The listing builds one solid part. Answer for the finished solid, in the listing's coordinates (mm). A direction names the side the tool comes from. Coordinates: 2 decimals unless noted, no trailing zeros. Order: outer loops, then holes, each group sorted by start corner. A loop starts at its lowest first (then second) coordinate and runs counter-clockwise, first axis right, second up. Notation, with made-up numbers: (80.25, -33) -> (119.25, -33) arc R9 cw to (119.25, -18) -> close; hole circle Ø10 at (83, 65). An arc over 180 degrees is marked (long way). Write item = value, one per line.
from build123d import *

# Parameters (mm, degrees)
SKETCH1_W               = 2.54
SKETCH1_H               = 6.35
SKETCH2_W               = 1.5875
SKETCH2_H               = 11.1125
CUT_EXTRUDE1_DEPTH      = 4.96875
CUT_EXTRUDE1_DEPTH_BACK = 4.96875


with BuildPart() as part:
    # Sketch1 → Revolve1 (revolve)
    with BuildSketch(Plane(origin=(0, 0, 0), x_dir=(0, 0, -1), z_dir=(1, 0, 0))):
        Polygon((0, 3.175), (0, 0), (3.96875, 0), (3.96875, 3.175), (2.54, 3.175), align=None)
        with Locations((1.27, 6.35)):
            Rectangle(SKETCH1_W, SKETCH1_H)
        Polygon((0, 14.2875), (0, 9.525), (2.54, 9.525), (3.175, 9.525), (1.5875, 14.2875), align=None)
    revolve(axis=Axis((0, 0, 0), (0, 1, 0)))

    # Sketch2 → Cut-Extrude1 (cut, two sides)
    with BuildSketch(Plane.XY) as cut_extrude1_sk:
        with Locations((0, 8.73125)):
            Rectangle(SKETCH2_W, SKETCH2_H)
    extrude(amount=CUT_EXTRUDE1_DEPTH, mode=Mode.SUBTRACT)
    extrude(cut_extrude1_sk.sketch, amount=-CUT_EXTRUDE1_DEPTH_BACK, mode=Mode.SUBTRACT)


solid = part.part
Q1. Each of these flat-tipped pins is pushed along its axis until it touches: pin 1 Ø3 at (x, z) = (0.5, 0.5) entering from -Y; pin 2 Ø3 at (x, y) = (-3, 1.5) entering from -Z; pin 3 Ø1.8 at (y, z) = (6.5, 1.5) entering from +X. Where does it stop, or does it pass through?
The answers:
pin_1 = 0
pin_2 = -3.67
pin_3 = 2.47
Q2. Section D-D, the plane z = 2.75 is taken. Give the number of separate pieces and of enclosed holes in the cut face, plus the area to 3 significant figures.
The answers:
separate_pieces = 3
enclosed_holes = 0
area = 19.0 mm2
Q3. A tool of negligible diameter and unlimited length cuts with its end or side. For faces 1 (the face through (-0.794, 9, 0)), 2 (the face through (-3, 9.525, 0)), 3 (the face through (2.37, 11.94, 0.04)), 4 (the face through (0, 3.175, 0)), 5 (the face through (3, 9.525, 0)), from which of +Z, -Z, +X, -X, +Y, -Y can it reach the whole face along a straight path? Write none if from no direction.
The answers:
face_1 = +Z, -Z, +Y
face_2 = -X
face_3 = +X, +Y
face_4 = none
face_5 = +X
Q4. Section A-A, the plane z = 0 is taken. Give the vertices of the cut face in (x, y) (1 decimal), plus the area to 3 significant figures.
The answers:
outline = (-4, 0) -> (4, 0) -> (4, 3.2) -> (2.5, 3.2) -> (2.5, 9.5) -> (3.2, 9.5) -> (1.6, 14.3) -> (0.8, 14.3) -> (0.8, 3.2) -> (-0.8, 3.2) -> (-0.8, 14.3) -> (-1.6, 14.3) -> (-3.2, 9.5) -> (-2.5, 9.5) -> (-2.5, 3.2) -> (-4, 3.2) -> close
area = 62.5 mm2
Q5. Find the intervals of material crossed by line 1 along X through (y, z) = (7.25, 1.75); line 2 along X through (y, z) = (9.25, -1.5); line 3 along Y through (x, z) = (0, -2.25) (3 decimals), in increasing order.
The answers:
line_1 = -1.84 to -0.79, 0.79 to 1.84
line_2 = -2.05 to -0.79, 0.79 to 2.05
line_3 = 0 to 3.175
Q6. Section C-C, the plane x = 0 is taken. Give the vertices of the cut face in (y, z) (3 decimals).
The answers:
outline = (0, -3.969) -> (3.175, -3.969) -> (3.175, 3.969) -> (0, 3.969) -> close
Q7. The mould has two halves that part along X. Classify faces 6 (the face through (0.794, 9, 0)), 7 (the face through (2.54, 6.39, 0.04)), 8 (the face through (3.874, 1.61, 0.86)): released by +X, released by -X, zero draft, split by the parting line, or undercut.
The answers:
face_6 = undercut
face_7 = released by +X
face_8 = split by the parting line
Q8. Section B-B, the plane y = 7 is taken. Give the vertices of the cut face in (x, z), plus the area to 3 significant figures.
The answers:
outline = (-0.79, -2.41) -> (-0.79, 2.41) arc R2.54 ccw to start; (0.79, -2.41) arc R2.54 ccw to (0.79, 2.41) -> close
area = 12.3 mm2
